```python
from build123d import *

# Parameters (mm, degrees)
SKETCH1_R           = 1.5
BOSS_EXTRUDE1_DEPTH = 3


with BuildPart() as part:
    # Sketch1 → Boss-Extrude1 (new body)
    with BuildSketch(Plane.XY):
        with BuildLine():
            Line((10.853563951, -24.90575827), (-10.853563951, -24.90575827))
            Line((-10.853563951, -24.90575827), (-4.723810622, 11.106542541))
            ThreePointArc((-4.723810622, 11.106542541), (-3.090959868, 13.964026902), (0, 15.09424173))
            ThreePointArc((0, 15.09424173), (3.090959868, 13.964026902), (4.723810622, 11.106542541))
            Line((4.723810622, 11.106542541), (10.853563951, -24.90575827))
        make_face()
        with Locations((0, 10.09424173)):
            Circle(SKETCH1_R, mode=Mode.SUBTRACT)
    extrude(amount=BOSS_EXTRUDE1_DEPTH)


solid = part.part
```
Geometry: final body of the model. Coordinates: model frame, mm. Give positions to 0.01 mm unless a question says otherwise; leave off trailing zeros. Write each loop counter-clockwise with the first axis right and the second up, starting at its lowest first coordinate (ties: lowest second). Pieces come first, ordered by that corner, then holes.
1. Section query C-C, the plane y = -14.5. Return loops of the section in (x, z), then the cut area to 3 significant figures.
2. Section query B-B, the plane z = 0.6. Return loops of the section in (x, y).
3. Section query D-D, the plane x = -3.75. Return loops of the section in (y, z).
4. Pin query (flat end, axial travel): P1, Ø2.5, axis at x = 0, y = 10.09, coming from the +Z side; P2, Ø1, axis at y = -1.5, z = 2, coming from the -X side; P3, Ø1, axis at y = -5.5, z = 1.5, coming from the +X side; P4, Ø5, axis at x = 5, y = -10.5, coming from the -Z side. Return the tip coordinate at first contact, or that it passes through.
5. Section query A-A, the plane x = 0.75. Return loops of the section in (y, z).
6. Draft query along X for faces 1 (the flat face through (0, -9, 3)), 2 (the cylindrical face through (-0.2, 11.58, 1.48)), 3 (the flat face through (-7.83, -7.15, 1.48)). Return one class per face: released by +X, released by -X, zero draft, split by the parting line, or undercut.
7. Line query: probe 1 along X at (y, z) = (13, 1.25); probe 2 along X at (y, z) = (-12.5, 0.75). Output: solid intervals per line, ascending.
Computed:
1. outline: (-9.08, 0) - (9.08, 0) - (9.08, 3) - (-9.08, 3) - close
1. area: 54.5 mm2
2. outline: (-10.85, -24.91) - (10.85, -24.91) - (4.72, 11.11) arc R4.79 ccw to (-4.72, 11.11) - close; hole circle Ø3 at (0, 10.09)
3. outline: (-24.91, 0) - (13.29, 0) - (13.29, 3) - (-24.91, 3) - close
4. P1: passes through
4. P2: stops at x = -6.95
4. P3: stops at x = 7.64
4. P4: stops at z = 0
5. outline: (-24.91, 0) - (8.8, 0) - (8.8, 3) - (-24.91, 3) - close; (11.39, 0) - (15.04, 0) - (15.04, 3) - (11.39, 3) - close
6. face 1: zero draft
6. face 2: undercut
6. face 3: released by -X
7. probe 1: x = -3.96 to 3.96
7. probe 2: x = -8.74 to 8.74
